Geometry check sheet. Reference: the model listing, model coordinates, mm. A direction names the side the tool comes from. Round coordinates to 2 decimals unless told otherwise and drop trailing zeros. Write each loop counter-clockwise with the first axis right and the second up, starting at its lowest first coordinate (ties: lowest second). Pieces come first, ordered by that corner, then holes.
from build123d import *

# Parameters (mm, degrees)
F0_R     = 5.5
F1_DEPTH = 0.1
F2_R     = 3.875
F3_DEPTH = 6
F4_DEPTH = 3
F5_R     = 4
F6_DEPTH = 7
F7_R     = 2.75
F7_R_2   = 1.05
F8_DEPTH = 15
F9_R     = 1


# Not quite as in the source:
# - a fillet or chamfer that OpenCascade refuses, or shapes differently, is made with other operations: its cross-section is extruded or revolved along the edge and cut away or added


with BuildPart() as f1:
    # F0 (on Top) → F1 (new body)
    with BuildSketch(Plane.XY):
        Circle(F0_R)
    extrude(amount=F1_DEPTH)

    # F2 (on face) → F3 (join)
    with BuildSketch(Plane.XY.offset(0.1)):
        Circle(F2_R)
    extrude(amount=F3_DEPTH)

    # F0 (on Top) → F4 (join)
    with BuildSketch(Plane.XY):
        Circle(F0_R)
    extrude(amount=-F4_DEPTH)

    # F5 (on face) → F6 (join)
    with BuildSketch(Plane(origin=(0, 0, -3), x_dir=(1, 0, 0), z_dir=(0, 0, -1))):
        Circle(F5_R)
    extrude(amount=F6_DEPTH)

    # F7 (on face) → F8 (cut)
    with BuildSketch(Plane.XY.offset(6.1)):
        Circle(F7_R)
        Circle(F7_R_2, mode=Mode.SUBTRACT)
    extrude(amount=-F8_DEPTH, mode=Mode.SUBTRACT)

    # F9
    f9_edges = [f1.edges().sort_by_distance(p)[0] for p in [
        (-1.05, 0, 6.1),
    ]]
    fillet(f9_edges, radius=F9_R)

    # F10: fillet of radius 2 on 1 edges, made by hand

    # F10_s1 → F10_t2 (revolve, cut)
    with BuildSketch(Plane.XZ):
        with BuildLine():
            ThreePointArc((5.5, -1.0635083269), (5.0811388301, -2.2882531983), (4, -3))
            Line((4, -3), (5.5, -3))
            Line((5.5, -3), (5.5, -1.0635083269))
        make_face()
    revolve(axis=Axis((0, 0, -3), (0, 0, 1)), mode=Mode.SUBTRACT)


solid = f1.part
1. Access from +Z, -Z, +X, -X, +Y, -Y to the whole of each face (thin tool, end or side, straight path). Record for faces 5 (the face through (1, -1, -8.9)), 6 (the face through (-3, -1, 6.1)).
2. Release check for a two-part mould opening along X. For faces 1 (the face through (1, 4, 0.1)), 2 (the face through (-0.867, 3.905, -6.451)), 3 (the face through (-0.596, -2.685, -1.295)), 4 (the face through (1, 0.32, -1.8)) record: +X half, -X half, draft (parallel to the pull), parting line (faces both ways), or undercut.
3. Scan lines: line 1 along Y through (x, z) = (0, -4.25); line 2 along Y through (x, z) = (0, -1); line 3 along X through (y, z) = (0.25, -3.5). Record each from-to range of solid material in increasing order.
4. Section check A-A (z = -1.75). Record the cut outline in (x, y), plus the area to 3 significant figures.
5. Depth check by flat-ended pin: pin 1 Ø1.5 at (x, z) = (-4, 3.5) entering from -Y; pin 2 Ø1.6 at (x, y) = (1.5, 0) entering from +Z; pin 3 Ø6 at (x, z) = (0, -7.5) entering from +Y. Enter the tip coordinate at first touch or a pass-through.
Results below:
1. face 5: +Z
1. face 6: +Z, +X, -X, +Y, -Y
2. face 1: draft
2. face 2: parting line
2. face 3: undercut
2. face 4: undercut
3. line 1: y = -4 to -2.75, -1.05 to 1.05, 2.75 to 4
3. line 2: y = -5.5 to -2.75, -1.05 to 1.05, 2.75 to 5.5
3. line 3: x = -3.99 to -2.74, -1.02 to 1.02, 2.74 to 3.99
4. outline: circle Ø10.76 at (0, 0); circle Ø2.1 at (0, 0); hole circle Ø5.5 at (0, 0)
4. area: 70.6 mm2
5. pin 1: stops at y = -2.11
5. pin 2: stops at z = 5.86
5. pin 3: stops at y = 4
